For this review, take the finished solid that the model builds, in its own axes (mm). A direction names the side the tool comes from. Give positions to 0.01 mm unless a question says otherwise; leave off trailing zeros. Write each loop counter-clockwise with the first axis right and the second up, starting at its lowest first coordinate (ties: lowest second). Pieces come first, ordered by that corner, then holes.
Q1. Insertion check: P1, Ø1, axis at x = 1, y = 3, coming from the -Z side; P2, Ø4, axis at y = -2.5, z = -5, coming from the +X side; P3, Ø1, axis at x = 1.5, y = -2, coming from the -Z side; P4, Ø1, axis at x = 2, y = 15, coming from the +Z side. Each pin has a flat end and moves straight along its axis. Give the tip position at first contact, or say it passes through.
Q2. Mouldability with a two-part tool opening along Y and no side actions: class faces 4 (the flat face through (1, -7.413, 5)), 5 (the flat face through (1.479, 10.717, 21.482)), 6 (the flat face through (1.479, 12.928, -9.534)) as released by +Y, released by -Y, zero draft, split by the parting line, or undercut.
Q3. We need section B-B (x = 1.85). Write out the cut boundary in (y, z).
Q4. We need section C-C (y = 9.5). Write out the cut boundary in (x, z), then the cut area to 3 significant figures.
Q5. Machinability: for faces 1 (the flat face through (1, -0.013, 6)), 2 (the flat face through (1.479, -2.785, 14.754)), 3 (the flat face through (0, -0.5, 7.6)), which of the approach directions +Z, -Z, +X, -X, +Y, -Y give a long, thin tool a straight path to every point of the face, cutting with its end or side? Answer none if there is none.
Q6. For line 1 (Y direction, x = 1.45, z = 0.5); line 2 (Z direction, x = 2.2, y = 11); line 3 (Z direction, x = 1.3, y = -3), list the stretches that pass through material, from the lowest coordinate up.
Q7. We need section D-D (z = 19). Write out the cut boundary in (x, y), then the cut area to 3 significant figures.
Q8. We need section A-A (z = 7.5). Write out the cut boundary in (x, y).
```python
from build123d import *

# Parameters (mm, degrees)
SKETCH1_W           = 26.4
SKETCH1_H           = 3.4
BOSS_EXTRUDE1_DEPTH = 3
CUT_EXTRUDE1_DEPTH  = 3


with BuildPart() as part:
    # Sketch1 → Boss-Extrude1 (new body)
    with BuildSketch(Plane(origin=(0, 0, 0), x_dir=(0, 0, -1), z_dir=(1, 0, 0))):
        Polygon((-29.192028343, 26.236188028), (-35.394898574, 22.200794504), (-16.635771919, -6.634169813), (-16.129107702, -7.412971773), (-15.2, -7.412971773), (15.2, -7.412971773), (15.2, -0.012971773), (-12.115145296, -0.012971773), align=None)
        with Locations((0, -3.712971773)):
            Rectangle(SKETCH1_W, SKETCH1_H, mode=Mode.SUBTRACT)
        Polygon((-13.30906469, -1.845326631), (-29.886897548, 23.636734858), (-32.736864952, 21.78263513), (-16.159032093, -3.699426359), align=None, mode=Mode.SUBTRACT)
    extrude(amount=BOSS_EXTRUDE1_DEPTH)

    # Sketch2 → Cut-Extrude1 (cut)
    with BuildSketch(Plane(origin=(3, 0, 0), x_dir=(0, 0, -1), z_dir=(1, 0, 0))):
        Polygon((15.2, -0.012971773), (-5.5, -0.012971773), (-5.5, -2.012971773), (13.2, -2.012971773), (13.2, -5.412971773), (-5.5, -5.412971773), (-5.5, -7.412971773), (15.2, -7.412971773), align=None)
    extrude(amount=-CUT_EXTRUDE1_DEPTH, mode=Mode.SUBTRACT)

    # Mirror1: part across plane


with BuildPart() as part_1:
    add(part.part)
    add(part.part.mirror(Plane.XY.offset(5.5)))


solid = part_1.part
```
Computed:
1. P1: stops at z = -12.23
1. P2: stops at x = 3
1. P3: stops at z = -8.98
1. P4: stops at z = 31.04
2. face 4: released by -Y
2. face 5: undercut
2. face 6: released by +Y
3. outline: (-7.41, -5.13) - (22.2, -24.39) - (26.24, -18.19) - (-0.01, -1.12) - (-0.01, 12.12) - (26.24, 29.19) - (22.2, 35.39) - (-7.41, 16.13) - close; hole (-5.41, -2.2) - (-2.01, -2.2) - (-2.01, 13.2) - (-5.41, 13.2) - close; hole (-3.7, -5.16) - (21.78, -21.74) - (23.64, -18.89) - (-1.85, -2.31) - close; hole (-3.7, 16.16) - (-1.85, 13.31) - (23.64, 29.89) - (21.78, 32.74) - close
4. outline: (0, -16.13) - (3, -16.13) - (3, -13.75) - (0, -13.75) - close; (0, -9.69) - (3, -9.69) - (3, -7.3) - (0, -7.3) - close; (0, 18.3) - (3, 18.3) - (3, 20.69) - (0, 20.69) - close; (0, 24.75) - (3, 24.75) - (3, 27.13) - (0, 27.13) - close
4. area: 28.6 mm2
5. face 1: +X, -X, +Y
5. face 2: +X, -X
5. face 3: +Z, -Z, -X, +Y, -Y
6. line 1: y = -7.41 to -5.41, -2.01 to -0.01
6. line 2: z = -17.11 to -14.72, -10.67 to -8.28, 19.28 to 21.67, 25.72 to 28.11
6. line 3: z = -8 to -5.61, -4.08 to -2.2, 13.2 to 15.08, 16.61 to 19
7. outline: (0, -3) - (3, -3) - (3, 0.67) - (0, 0.67) - close; (0, 6.9) - (3, 6.9) - (3, 10.57) - (0, 10.57) - close
7. area: 22.0 mm2
8. outline: (0, -7.41) - (3, -7.41) - (3, -5.41) - (0, -5.41) - close; (0, -2.01) - (3, -2.01) - (3, -0.01) - (0, -0.01) - close
